Autodesk Inventor part; units mm, degrees
ref_plane "YZ Plane" through (0, 0, 0) normal (1, 0, 0) x (0, 1, 0)
ref_plane "XZ Plane" through (0, 0, 0) normal (0, 1, 0) x (-1, 0, 0)
ref_plane "XY Plane" through (0, 0, 0) normal (0, 0, 1) x (1, 0, 0)
sketch "Sketch1" plane through (0, 0, 0) normal (0, 0, 1) x (1, 0, 0)
  circle A0 centre (0, 0) radius 2.5
  line L0 (-4.5, 5) -> (4.5, 5)
  line L1 (4.5, 5) -> (4.5, -11.5)
  line L2 (4.5, -11.5) -> (-4.5, -11.5)
  line L3 (-4.5, -11.5) -> (-4.5, 5)
  line L4 (-4.5, -11.5) -> (4.5, -11.5)
  line L5 (4.5, -11.5) -> (4.5, -15)
  line L6 (4.5, -15) -> (-4.5, -15)
  line L7 (-4.5, -15) -> (-4.5, -11.5)
  dimension "d0" = 5
  dimension "d1" = 4.5
  dimension "d2" = 4.5
  dimension "d3" = 5
  dimension "d4" = 11.5
  dimension "d5" = 3.5
extrude "Extrusion1" add sketch "Sketch1" along normal blind 3
sketch "Sketch2" plane through (0, 0, 3) normal (0, 0, 1) x (1, 0, 0)
  line L0 (4.5, 5) -> (-4.5, 5)
  line L1 (-4.5, 5) -> (-4.5, -15)
  line L2 (-4.5, -15) -> (4.5, -15)
  line L3 (4.5, -15) -> (4.5, 5)
  circle A0 centre (0, 0) radius 2.5
  line L4 (-4.5, -15) -> (4.5, -15)
  line L5 (4.5, -15) -> (4.5, -11.5)
  line L6 (4.5, -11.5) -> (-4.5, -11.5)
  line L7 (-4.5, -11.5) -> (-4.5, -15)
  dimension "d8" = 3.5
extrude "Extrusion2" add sketch "Sketch2" along normal blind 10 contours L3 L2 L1 L6
sketch "Sketch3" plane through (-4.5, -11.5, 3) normal (0, 1, 0) x (1, 0, 0)
  point P0 (4.5, 3)
  point P1 (4.4515, -6.2435)
hole "Hole1" at (-0.0485, -11.5, 9.2435) direction (0, -1, 0) diameter 5.5 depth 4 tip angle 118
fillet "Fillet1" radius 1.25 5 edges at (4.5, -13.25, 13) (-4.5, -13.25, 13) (0, -11.5, 3) (4.5, 5, 1.5) (-4.5, 5, 1.5)
properties part number "driver-bracket_3DPrint"
The listing builds one solid part. Answer for the finished solid, in the listing's coordinates (mm). A direction names the side the tool comes from. Give positions to 0.01 mm unless a question says otherwise; leave off trailing zeros. Order: outer loops, then holes, each group sorted by start corner. A loop starts at its lowest first (then second) coordinate and runs counter-clockwise, first axis right, second up. Notation, with made-up numbers: (11, -3.5) -> (61, -3.5) arc R35 ccw to (61, 34.5) -> close; hole circle Ø9 at (9.25, 24). An arc over 180 degrees is marked (long way). Answer as a JSON object with one key per item and string values. Group by question number.
Item 1: The part is cut by section B-B on z = 7.25. Write down the section's boundary in (x, y), and give its area (3 significant figures).
Item 2: Determine the mould class of faces 3 (the flat face through (0, -5, 0)), 4 (the cylindrical face through (-0.87, -13.27, 11.87)), 5 (the cylindrical face through (4.144, 4.624, 1.521)), 6 (the cylindrical face through (4.124, -13.226, 12.644)) for opening direction Z: pulls with the +Z half, pulls with the -Z half, needs draft (parallel to the pull), parting line crosses it, or undercut.
Item 3: The part is cut by section D-D on z = 1.75. Write down the section's boundary in (x, y).
Item 4: Flat-ended cylindrical pins translate along their axes: pin 1 (2 mm diameter, centred on x = 2.5, y = -2, fed in from -Z); pin 2 (4.5 mm diameter, centred on x = 1, z = 10.5, fed in from +Y); pin 3 (3 mm diameter, centred on x = -1, y = -7, fed in from +Z); pin 4 (1.5 mm diameter, centred on x = 1, y = -1, fed in from +Z). Find the tip coordinate at first contact, or state that the pin passes through.
Item 5: Consider L1, parallel to Y at x = 0, z = 1.8; L2, parallel to Y at x = 0.25, z = 6; L3, parallel to Z at x = -1, y = -12. Determine where each line is inside the solid, lowest interval first. Write a range as from..to.
Item 6: A tool of negligible diameter and unlimited length cuts with its end or side. For faces 1 (the flat face through (0, -3, 3)), 2 (the flat face through (0, -13, 13)), from which of +Z, -Z, +X, -X, +Y, -Y can it reach the whole face along a straight path? Write none if from no direction.
Item 7: The part is cut by section C-C on x = 1.5. Write down the section's boundary in (y, z).
Item 8: The part is cut by section A-A on y = 0. Write down the section's boundary in (x, z), and give its area (3 significant figures).
Result set:
{
 "1": {"outline": "(-4.5, -15) -> (-1.94, -15) -> (-1.94, -11.5) -> (-4.5, -11.5) -> close; (1.85, -15) -> (4.5, -15) -> (4.5, -11.5) -> (1.85, -11.5) -> close", "area": "18.2 mm²"},
 "2": {"face 3": "pulls with the -Z half", "face 4": "undercut", "face 5": "needs draft", "face 6": "pulls with the +Z half"},
 "3": {"outline": "(-4.5, -15) -> (4.5, -15) -> (4.5, 3.75) arc R1.25 ccw to (3.25, 5) -> (-3.25, 5) arc R1.25 ccw to (-4.5, 3.75) -> close; hole circle Ø5 at (0, 0)"},
 "4": {"pin 1": "z = 0", "pin 2": "y = -11.5", "pin 3": "z = 3", "pin 4": "through"},
 "5": {"L1": "-15..-2.5, 2.5..5", "L2": "-15..-11.5", "L3": "0..6.66, 11.82..13"},
 "6": {"face 1": "+Z, +X, -X, +Y", "face 2": "+Z, +X, -X, +Y, -Y"},
 "7": {"outline": "(-15, 0) -> (-2, 0) -> (-2, 3) -> (-10.25, 3) arc R1.25 cw to (-11.5, 4.25) -> (-11.5, 6.97) -> (-15, 6.97) -> close; (-15, 11.52) -> (-11.5, 11.52) -> (-11.5, 13) -> (-15, 13) -> close; (2, 0) -> (5, 0) -> (5, 3) -> (2, 3) -> close"},
 "8": {"outline": "(-4.5, 0) -> (-2.5, 0) -> (-2.5, 3) -> (-4.5, 3) -> close; (2.5, 0) -> (4.5, 0) -> (4.5, 3) -> (2.5, 3) -> close", "area": "12.0 mm²"}
}
